Drawing for the job (mm, zero at the part's lowest x, y, z). Give positions to 0.01 mm unless a question says otherwise; leave off trailing zeros. Use a Markdown table: item, result.
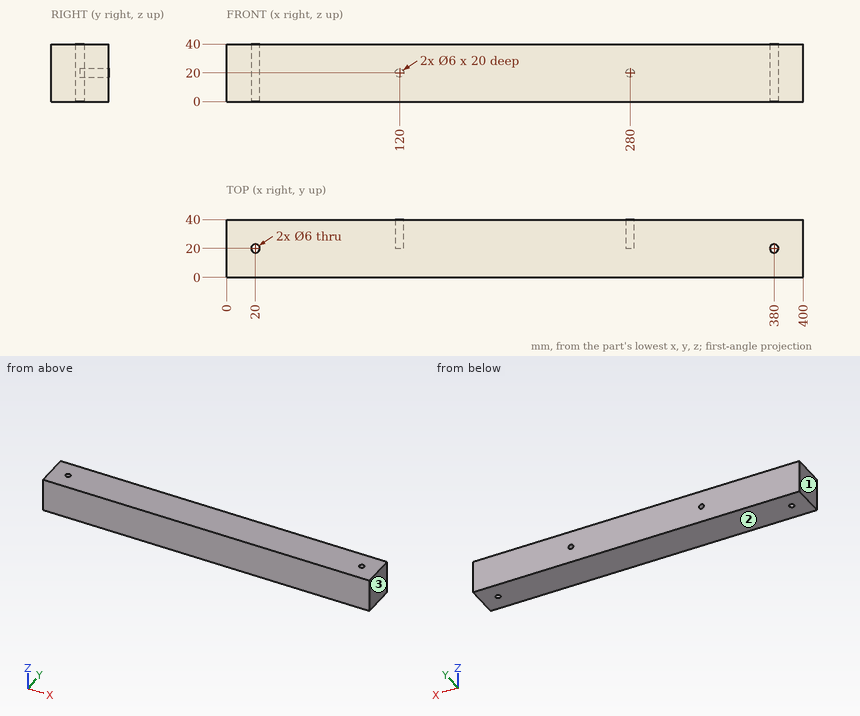
1) Two-plate mould, pull along X, no slides. Class the marked faces 1, 2 and 3: +X half, -X half, draft (parallel to the pull), parting line (faces both ways), or undercut.
Computed:
| item | result |
|---|---|
| face 1 | -X half |
| face 2 | draft |
| face 3 | +X half |
2) Pin check, flat tip, straight feed: P1, Ø1.8, axis at x = 119.5, z = 19.5, coming from the +Y side. Stop position of the tip, or through.
Computed:
| item | result |
|---|---|
| P1 | stops at y = 20 |
3) Wall check: line 1 (Y direction, x = 20, z = 30). Give the ranges that are in metal, low to high. Write a range as from..to.
Computed:
| item | result |
|---|---|
| line 1 | y = 0..17, 23..40 |
